from build123d import *

# Parameters (mm, degrees)
SKETCH1_W           = 121.6
SKETCH1_H           = 44.82
BOSS_EXTRUDE1_DEPTH = 3
CUT_EXTRUDE1_REACH  = 5
SKETCH4_W           = 42
SKETCH4_H           = 22
SKETCH5_W           = 3
SKETCH5_H           = 8.964
CUT_EXTRUDE2_DEPTH  = 4


with BuildPart() as part:
    # Sketch1 → Boss-Extrude1 (new body)
    with BuildSketch(Plane.XY):
        with Locations((60.8, 22.41)):
            Rectangle(SKETCH1_W, SKETCH1_H)
    extrude(amount=BOSS_EXTRUDE1_DEPTH)

    # Sketch4 → Cut-Extrude1 (cut, up to next)
    with BuildSketch(Plane.XY.offset(3), mode=Mode.PRIVATE) as cut_extrude1_sk1:
        with Locations((94.6, 30.82)):
            Rectangle(SKETCH4_W, SKETCH4_H)
    cut_extrude1_tool1 = extrude(cut_extrude1_sk1.sketch, amount=-CUT_EXTRUDE1_REACH, mode=Mode.PRIVATE) & part.part
    add(cut_extrude1_tool1.solids().sort_by_distance((94.6, 30.82, 3))[0], mode=Mode.SUBTRACT)

    # Sketch5 → Cut-Extrude2 (cut, through all)
    with BuildSketch(Plane.XY.offset(3)):
        with Locations((1.5, 13.446)):
            Rectangle(SKETCH5_W, SKETCH5_H)
        with Locations((1.5, 31.374)):
            Rectangle(SKETCH5_W, SKETCH5_H)
        with Locations((120.1, 13.446)):
            Rectangle(SKETCH5_W, SKETCH5_H)
        with Locations((120.1, 31.374)):
            Rectangle(SKETCH5_W, SKETCH5_H)
    extrude(amount=-CUT_EXTRUDE2_DEPTH, mode=Mode.SUBTRACT)


solid = part.part
For this review, take the finished solid that the model builds, in its own axes (mm). A direction names the side the tool comes from. Coordinates: 2 decimals unless noted, no trailing zeros. Loops run counter-clockwise (first coordinate to the right, second up) from the corner with the lowest first, then second, coordinate; pieces in that order, holes last. Notation, with made-up numbers: (18, 78) - (32, 78) arc R18 cw to (32, 87) - close; hole circle Ø1 at (5, 48). An arc over 180 degrees is marked (long way). Return JSON: item names as keys, results as strings.
Item 1: For line 1 (Y direction, x = 87.5, z = 1); line 2 (X direction, y = 32, z = 2.55); line 3 (X direction, y = 22, z = 1.45), list the stretches that pass through material, from the lowest coordinate up.
Determined:
{"line 1": "y = 0 to 19.82, 41.82 to 44.82", "line 2": "x = 3 to 73.6, 115.6 to 118.6", "line 3": "x = 0 to 73.6, 115.6 to 121.6"}
Item 2: Mouldability with a two-part tool opening along X and no side actions: class faces 4 (the flat face through (121.6, 4, 1)), 5 (the flat face through (94, 41.82, 2)), 6 (the flat face through (120, 8.964, 2)) as pulls with the +X half, pulls with the -X half, needs draft (parallel to the pull), parting line crosses it, or undercut.
Determined:
{"face 4": "pulls with the +X half", "face 5": "undercut", "face 6": "needs draft"}
Item 3: Take a section at B-B (x = 80.5). Give the boundary of the cut face in (y, z), then the cut area to 3 significant figures.
Determined:
{"outline": "(0, 0) - (19.82, 0) - (19.82, 3) - (0, 3) - close; (41.82, 0) - (44.82, 0) - (44.82, 3) - (41.82, 3) - close", "area": "68.5 mm2"}
Item 4: For faces 1 (the flat face through (118.6, 13, 2)), 2 (the flat face through (73.6, 31, 2)), 3 (the flat face through (3, 31, 2)), list the 3-axis set-ups (+Z, -Z, +X, -X, +Y, -Y) from which the entire face can be reached by the end or side of a thin tool; tool diameter is ignored.
Determined:
{"face 1": "+Z, -Z, +X", "face 2": "+Z, -Z", "face 3": "+Z, -Z, -X"}
Item 5: Take a section at C-C (y = 23). Give the boundary of the cut face in (x, z).
Determined:
{"outline": "(0, 0) - (73.6, 0) - (73.6, 3) - (0, 3) - close; (115.6, 0) - (121.6, 0) - (121.6, 3) - (115.6, 3) - close"}
Item 6: Take a section at A-A (z = 1.7). Give the boundary of the cut face in (x, y), then the cut area to 3 significant figures.
Determined:
{"outline": "(0, 0) - (121.6, 0) - (121.6, 8.96) - (118.6, 8.96) - (118.6, 17.93) - (121.6, 17.93) - (121.6, 26.89) - (118.6, 26.89) - (118.6, 35.86) - (121.6, 35.86) - (121.6, 44.82) - (0, 44.82) - (0, 35.86) - (3, 35.86) - (3, 26.89) - (0, 26.89) - (0, 17.93) - (3, 17.93) - (3, 8.96) - (0, 8.96) - close; hole (73.6, 19.82) - (115.6, 19.82) - (115.6, 41.82) - (73.6, 41.82) - close", "area": "4,420 mm2"}
Item 7: Insertion check: pin 1 (1.5 mm diameter, centred on y = 33.5, z = 1, fed in from -X). The pin has a flat end and moves straight along its axis. Give the tip position at first contact, or say it passes through.
Determined:
{"pin 1": "stops at x = 3"}
Item 8: Take a section at D-D (y = 16). Give the boundary of the cut face in (x, z), then the cut area to 3 significant figures.
Determined:
{"outline": "(3, 0) - (118.6, 0) - (118.6, 3) - (3, 3) - close", "area": "347 mm2"}
